```python
from build123d import *

# Parameters (mm, degrees)
SKETCH1_R           = 2.15
BOSS_EXTRUDE1_DEPTH = 5.461
FILLET1_R           = 10
SKETCH2_W           = 4.7625
SKETCH2_H           = 33.783
CUT_EXTRUDE1_DEPTH  = 10


with BuildPart() as part:
    # Sketch1 → Boss-Extrude1 (new body)
    with BuildSketch(Plane(origin=(0, 0, 0), x_dir=(1, 0, 0), z_dir=(0, 1, 0))):
        Polygon((0, 0), (-92, 92), (-92, 110), (-56.601944845, 110), (0, 94.833554589), (0, 58.293), (8, 58.293), (8, -58.293), (0, -58.293), (0, -94.833554589), (-56.601944845, -110), (-92, -110), (-92, -92), align=None)
        with Locations((-85.159917522, 94.147890435)):
            Circle(SKETCH1_R, mode=Mode.SUBTRACT)
        with Locations((-81.358825255, 103.397306502)):
            Circle(SKETCH1_R, mode=Mode.SUBTRACT)
        with Locations((-36.961628134, 85.152063619)):
            Circle(SKETCH1_R, mode=Mode.SUBTRACT)
        with Locations((-40.762720402, 75.902647552)):
            Circle(SKETCH1_R, mode=Mode.SUBTRACT)
        with Locations((-40.762720402, -75.902647552)):
            Circle(SKETCH1_R, mode=Mode.SUBTRACT)
        with Locations((-36.961628134, -85.152063619)):
            Circle(SKETCH1_R, mode=Mode.SUBTRACT)
        with Locations((-81.358825255, -103.397306502)):
            Circle(SKETCH1_R, mode=Mode.SUBTRACT)
        with Locations((-85.159917522, -94.147890435)):
            Circle(SKETCH1_R, mode=Mode.SUBTRACT)
        with BuildLine():
            Line((-79.322036695, 97.830250065), (-76.328676535, 105.114165218))
            ThreePointArc((-76.328676535, 105.114165218), (-76.087243425, 105.511850251), (-75.735570504, 105.816431091))
            ThreePointArc((-75.735570504, 105.816431091), (-75.067221358, 106.038703614), (-74.371100284, 105.931413788))
            Line((-74.371100284, 105.931413788), (-40.148260837, 91.867372399))
            ThreePointArc((-40.148260837, 91.867372399), (-39.577853455, 91.454176231), (-39.258927152, 90.826178087))
            ThreePointArc((-39.258927152, 90.826178087), (-39.223044121, 90.362329254), (-39.331012268, 89.909796149))
            Line((-39.331012268, 89.909796149), (-42.324372428, 82.625880996))
            Line((-42.324372428, 82.625880996), (-36.219757824, 80.1171601))
            Line((-36.219757824, 80.1171601), (-36.694894357, 78.960983092))
            Line((-36.694894357, 78.960983092), (-42.799508961, 81.469703988))
            Line((-42.799508961, 81.469703988), (-45.792869122, 74.185788836))
            ThreePointArc((-45.792869122, 74.185788836), (-46.034302231, 73.788103802), (-46.385975153, 73.483522962))
            ThreePointArc((-46.385975153, 73.483522962), (-47.054324299, 73.261250439), (-47.750445372, 73.368540266))
            Line((-47.750445372, 73.368540266), (-81.973284819, 87.432581654))
            ThreePointArc((-81.973284819, 87.432581654), (-82.543692202, 87.845777823), (-82.862618505, 88.473775966))
            ThreePointArc((-82.862618505, 88.473775966), (-82.898501536, 88.937624799), (-82.790533389, 89.390157905))
            Line((-82.790533389, 89.390157905), (-79.797173228, 96.674073057))
            Line((-79.797173228, 96.674073057), (-85.901787832, 99.182793954))
            Line((-85.901787832, 99.182793954), (-85.426651299, 100.338970962))
            Line((-85.426651299, 100.338970962), (-79.322036695, 97.830250065))
        make_face(mode=Mode.SUBTRACT)
        with BuildLine():
            Line((-47.750445372, -73.368540266), (-81.973284819, -87.432581654))
            ThreePointArc((-81.973284819, -87.432581654), (-82.543692202, -87.845777823), (-82.862618505, -88.473775966))
            ThreePointArc((-82.862618505, -88.473775966), (-82.898501536, -88.937624799), (-82.790533389, -89.390157905))
            Line((-82.790533389, -89.390157905), (-79.797173228, -96.674073057))
            Line((-79.797173228, -96.674073057), (-85.901787832, -99.182793954))
            Line((-85.901787832, -99.182793954), (-85.426651299, -100.338970962))
            Line((-85.426651299, -100.338970962), (-79.322036695, -97.830250065))
            Line((-79.322036695, -97.830250065), (-76.328676535, -105.114165218))
            ThreePointArc((-76.328676535, -105.114165218), (-76.087243425, -105.511850251), (-75.735570504, -105.816431091))
            ThreePointArc((-75.735570504, -105.816431091), (-75.067221358, -106.038703614), (-74.371100284, -105.931413788))
            Line((-74.371100284, -105.931413788), (-40.148260837, -91.867372399))
            ThreePointArc((-40.148260837, -91.867372399), (-39.577853455, -91.454176231), (-39.258927152, -90.826178087))
            ThreePointArc((-39.258927152, -90.826178087), (-39.223044121, -90.362329254), (-39.331012268, -89.909796149))
            Line((-39.331012268, -89.909796149), (-42.324372428, -82.625880996))
            Line((-42.324372428, -82.625880996), (-36.219757824, -80.1171601))
            Line((-36.219757824, -80.1171601), (-36.694894357, -78.960983092))
            Line((-36.694894357, -78.960983092), (-42.799508961, -81.469703988))
            Line((-42.799508961, -81.469703988), (-45.792869122, -74.185788836))
            ThreePointArc((-45.792869122, -74.185788836), (-46.034302231, -73.788103802), (-46.385975153, -73.483522962))
            ThreePointArc((-46.385975153, -73.483522962), (-47.054324299, -73.261250439), (-47.750445372, -73.368540266))
        make_face(mode=Mode.SUBTRACT)
    extrude(amount=BOSS_EXTRUDE1_DEPTH)

    # Fillet1
    fillet1_edges = [part.edges().sort_by_distance(p)[0] for p in [
        (-92, 2.7305, -110),
        (-92, 2.7305, 110),
    ]]
    fillet(fillet1_edges, radius=FILLET1_R)

    # Sketch2 → Cut-Extrude1 (cut)
    with BuildSketch(Plane(origin=(0, 0, 0), x_dir=(1, 0, 0), z_dir=(0, 1, 0))):
        Polygon((-4.829629131, 96.127649814), (-17.19282542, 99.440358276), (-18.425451123, 94.840136528), (-6.062254834, 91.527428067), align=None)
        Polygon((-24.920232031, 101.510910637), (-37.283428319, 104.823619098), (-38.516054022, 100.22339735), (-26.152857733, 96.910688889), align=None)
        Polygon((-26.152857733, -96.910688889), (-38.516054022, -100.22339735), (-37.283428319, -104.823619098), (-24.920232031, -101.510910637), align=None)
        Polygon((-6.062254834, -91.527428067), (-18.425451123, -94.840136528), (-17.19282542, -99.440358276), (-4.829629131, -96.127649814), align=None)
        with Locations((5.61875, 33.4015)):
            Rectangle(SKETCH2_W, SKETCH2_H)
        with Locations((5.61875, -33.4015)):
            Rectangle(SKETCH2_W, SKETCH2_H)
    extrude(amount=CUT_EXTRUDE1_DEPTH, mode=Mode.SUBTRACT)


solid = part.part
```
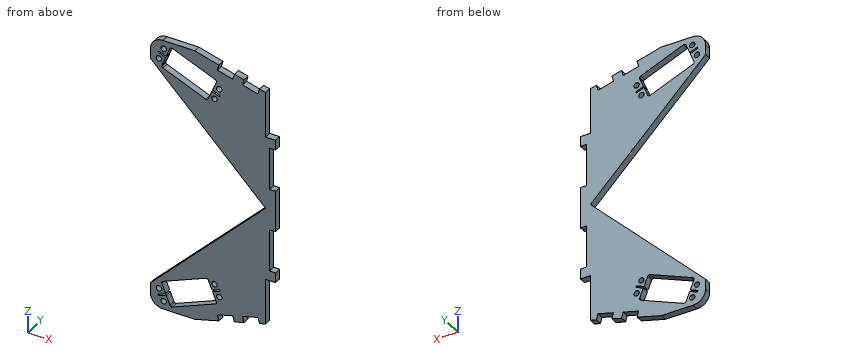
Check sheet for the modelled part. Datum: model origin and axes. Units: mm. Give positions to 0.01 mm unless a question says otherwise; leave off trailing zeros. Write each loop counter-clockwise with the first axis right and the second up, starting at its lowest first coordinate (ties: lowest second). Pieces come first, ordered by that corner, then holes.
Item 1: Cross-section at D-D (y = 4.1). Count the separate pieces of the cut face and the enclosed holes in it, and give its area (3 significant figures).
Item 2: Cross-section at A-A (x = -22). Enter the section's corners in (y, z).
Item 3: Scan lines: L1, parallel to Z at x = -61.5, y = 1.2; L2, parallel to X at y = 1.7, z = -86.5; L3, parallel to Z at x = -54.5, y = 3.9. Record each from-to range of solid material in increasing order.
Item 4: Cross-section at B-B (x = -53). Enter the section's corners in (y, z).
Item 5: Cross-section at C-C (z = 41). Enter the section's corners in (x, y).
Item 6: Gauge pin test, flat ends, axial feed: pin 1 (1 mm diameter, centred on y = 3.5, z = 31, fed in from -X); pin 2 (1.4 mm diameter, centred on x = 6, y = 3, fed in from +Z); pin 3 (1 mm diameter, centred on x = -23, y = 4.5, fed in from -Z). Record the tip position at first contact, or that the pin passes through.
Report:
1. separate pieces: 1
1. enclosed holes: 10
1. area: 9,500 mm2
2. outline: (0, -100.73) - (5.46, -100.73) - (5.46, -22) - (0, -22) - close; (0, 22) - (5.46, 22) - (5.46, 100.73) - (0, 100.73) - close
3. L1: z = -110 to -100.64, -79.02 to -61.5, 61.5 to 79.02, 100.64 to 110
3. L2: x = -86.5 to -79.7, -40.73 to -38.64, -35.29 to 0
3. L3: z = -109.44 to -97.77, -76.14 to -54.5, 54.5 to 76.14, 97.77 to 109.44
4. outline: (0, -109.03) - (5.46, -109.03) - (5.46, -97.15) - (0, -97.15) - close; (0, -75.53) - (5.46, -75.53) - (5.46, -53) - (0, -53) - close; (0, 53) - (5.46, 53) - (5.46, 75.53) - (0, 75.53) - close; (0, 97.15) - (5.46, 97.15) - (5.46, 109.03) - (0, 109.03) - close
5. outline: (-41, 0) - (3.24, 0) - (3.24, 5.46) - (-41, 5.46) - close
6. pin 1: stops at x = -31.5
6. pin 2: stops at z = 58.29
6. pin 3: stops at z = -101.13
